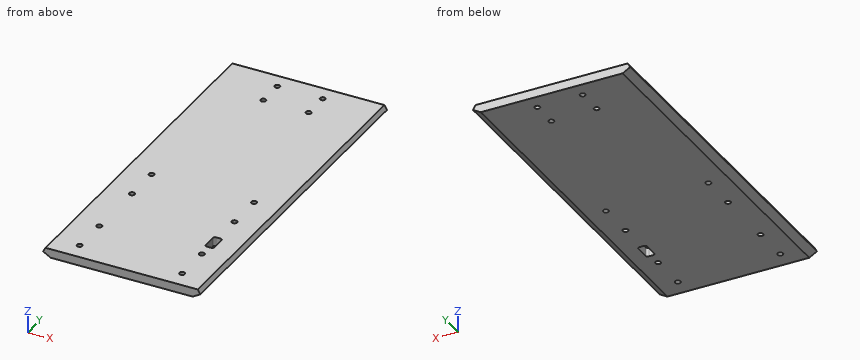
from build123d import *

# Parameters (mm, degrees)
SKETCH1_W           = 101.6
SKETCH1_H           = 254
BOSS_EXTRUDE1_DEPTH = 6.35
BOSS_EXTRUDE2_DEPTH = 254
CUT_EXTRUDE2_DEPTH  = 255
SKETCH5_R           = 1.905
CUT_EXTRUDE3_DEPTH  = 7.35
SKETCH6_R           = 1.905
CUT_EXTRUDE4_DEPTH  = 7.35
SKETCH9_W           = 6.35
SKETCH9_H           = 12.7
CUT_EXTRUDE5_DEPTH  = 7.35
FILLET1_R           = 1.5875


with BuildPart() as part:
    # Sketch1 → Boss-Extrude1 (new body)
    with BuildSketch(Plane.XY):
        with Locations((0, -25.4)):
            Rectangle(SKETCH1_W, SKETCH1_H)
    extrude(amount=BOSS_EXTRUDE1_DEPTH)

    # Sketch2 → Boss-Extrude2 (add)
    with BuildSketch(Plane(origin=(0, 101.6, 0), x_dir=(1, 0, 0), z_dir=(0, 1, 0))):
        Polygon((-50.8, 0), (-61.798522628, -6.35), (-50.8, -6.35), align=None)
        Polygon((61.798522628, -6.35), (50.8, -6.35), (50.8, 0), align=None)
    extrude(amount=-BOSS_EXTRUDE2_DEPTH)

    # Sketch4 → Cut-Extrude2 (cut, through all)
    with BuildSketch(Plane(origin=(0, 101.6, 0), x_dir=(1, 0, 0), z_dir=(0, 1, 0))):
        Polygon((56.299261314, -3.175), (54.466174209, -6.35), (61.798522628, -6.35), align=None)
        Polygon((-61.798522628, -6.35), (-54.466174209, -6.35), (-56.299261314, -3.175), align=None)
    extrude(amount=-CUT_EXTRUDE2_DEPTH, mode=Mode.SUBTRACT)

    # Sketch5 → Cut-Extrude3 (cut, through all)
    with BuildSketch(Plane.XY.offset(6.35)):
        with Locations((-36.686174209, -41.91)):
            Circle(SKETCH5_R)
        with Locations((36.686174209, -41.91)):
            Circle(SKETCH5_R)
        with Locations((36.686174209, -68.58)):
            Circle(SKETCH5_R)
        with Locations((36.686174209, -113.03)):
            Circle(SKETCH5_R)
        with Locations((36.686174209, -139.7)):
            Circle(SKETCH5_R)
        with Locations((-36.686174209, -139.7)):
            Circle(SKETCH5_R)
        with Locations((-36.686174209, -113.03)):
            Circle(SKETCH5_R)
        with Locations((-36.686174209, -68.58)):
            Circle(SKETCH5_R)
    extrude(amount=-CUT_EXTRUDE3_DEPTH, mode=Mode.SUBTRACT)

    # Sketch6 → Cut-Extrude4 (cut, through all)
    with BuildSketch(Plane.XY.offset(6.35)):
        with Locations((-16.256, 90.17)):
            Circle(SKETCH6_R)
        with Locations((16.256, 90.17)):
            Circle(SKETCH6_R)
        with Locations((16.256, 71.12)):
            Circle(SKETCH6_R)
        with Locations((-16.256, 71.12)):
            Circle(SKETCH6_R)
    extrude(amount=-CUT_EXTRUDE4_DEPTH, mode=Mode.SUBTRACT)

    # Sketch9 → Cut-Extrude5 (cut, through all)
    with BuildSketch(Plane.XY.offset(6.35)):
        with Locations((36.813174209, -97.155)):
            Rectangle(SKETCH9_W, SKETCH9_H)
    extrude(amount=-CUT_EXTRUDE5_DEPTH, mode=Mode.SUBTRACT)

    # Fillet1
    fillet1_edges = [part.edges().sort_by_distance(p)[0] for p in [
        (33.638174209, -90.805, 3.175),
        (39.988174209, -90.805, 3.175),
        (39.988174209, -103.505, 3.175),
        (33.638174209, -103.505, 3.175),
    ]]
    fillet(fillet1_edges, radius=FILLET1_R)


solid = part.part
The model under review builds one solid part; all positions refer to its coordinate system, in mm. Round coordinates to 2 decimals unless told otherwise and drop trailing zeros. Write each loop counter-clockwise with the first axis right and the second up, starting at its lowest first coordinate (ties: lowest second). Pieces come first, ordered by that corner, then holes. Notation, with made-up numbers: M 27,16.5 L 48,16.5 A23 cw 48,46.5 Z; hole C 61.25,26 d5. An arc over 180 degrees is marked long. Use a Markdown table: item, result. Add a question column.
Q1. We need section B-B, the plane y = -52. State the section outline as (x, z) points (3 decimals).
Q2. We need section A-A, the plane z = 5.25. Count the separate pieces of the cut face and the enclosed holes in it, plus the area to 3 significant figures.
Q3. Insertion check: pin 1 (1.9 mm diameter, centred on y = -98.5, z = 2, fed in from -X); pin 2 (5 mm diameter, centred on x = -36.69, y = -68.58, fed in from -Z). Each pin has a flat end and moves straight along its axis. Give the tip position at first contact, or say it passes through.
Q4. To check wall thickness, follow line 1 (Y direction, x = 16.5, z = 1.75); line 2 (Y direction, x = -36.5, z = 5.25); line 3 (Y direction, x = 35, z = 4.5). State the ranges of each line that lie inside material, in increasing order.
Findings below:
| question | item | result |
|---|---|---|
| 1 | outline | M -56.299,3.175 L -50.8,0 L 50.8,0 L 56.299,3.175 L 54.466,6.35 L -54.466,6.35 Z |
| 2 | separate pieces | 1 |
| 2 | enclosed holes | 13 |
| 2 | area | 27,800 mm² |
| 3 | pin 1 | stops at x = -55.91 |
| 3 | pin 2 | stops at z = 0 |
| 4 | line 1 | y = -152.4 to 69.23, 73.01 to 88.28, 92.06 to 101.6 |
| 4 | line 2 | y = -152.4 to -141.6, -137.8 to -114.93, -111.13 to -70.48, -66.68 to -43.81, -40.01 to 101.6 |
| 4 | line 3 | y = -152.4 to -140.59, -138.81 to -113.92, -112.14 to -103.49, -90.82 to -69.47, -67.69 to -42.8, -41.02 to 101.6 |
